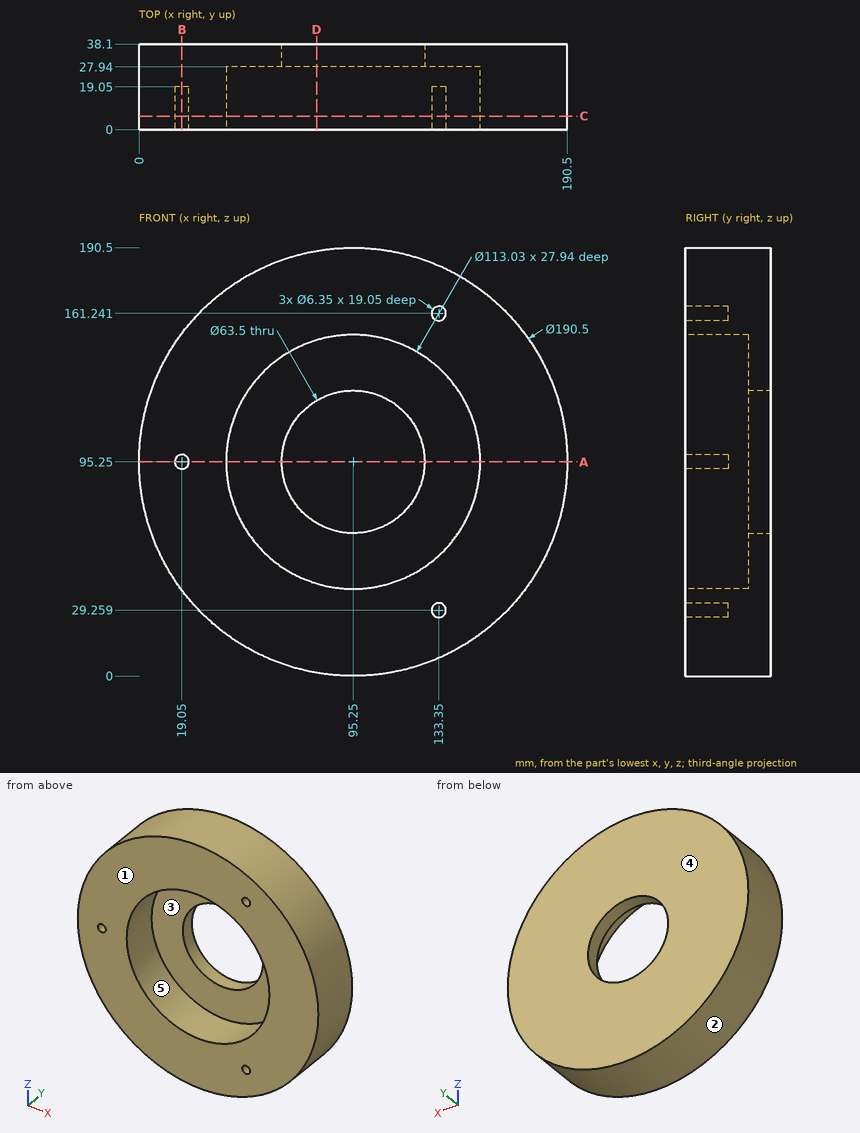
Source: three-view drawing plus pictorial views. Frame: mm from the lowest corner of the part. A direction names the side the tool comes from. Give positions to 0.01 mm unless a question says otherwise; leave off trailing zeros. Order: outer loops, then holes, each group sorted by start corner. A loop starts at its lowest first (then second) coordinate and runs counter-clockwise, first axis right, second up. Notation, with made-up numbers: (86.5, -36) - (118.5, -36) arc R27 cw to (118.5, -8) - close; hole circle Ø8 at (27.5, -23). An arc over 180 degrees is marked (long way). Answer as a JSON object with one key per item and string values. Group by question number.
Q1. Cut plane B-B, the plane x = 19.05. Output: boundary loops of the cut face in (y, z) (3 decimals).
Q2. Cut plane C-C, the plane y = 6. Count the separate pieces of the cut face and the enclosed holes in it, then the cut area to 3 significant figures.
Q3. Cut plane A-A, the plane z = 95.25. Output: boundary loops of the cut face in (x, y) (3 decimals).
Q4. Line query: probe 1 along X at (y, z) = (13, 95) (1 decimal); probe 2 along Z at (x, y) = (95.25, 33); probe 3 along Z at (x, y) = (133.35, 13.5). Output: solid intervals per line, ascending.
Q5. First-contact query: pin 1 Ø1.9 at (x, z) = (17.5, 95) entering from -Y; pin 2 Ø2 at (x, y) = (75, 16.5) entering from +Z; pin 3 Ø6 at (y, z) = (33.5, 28.5) entering from -X. Flat tips, straight axial feed; report the tip coordinate or a pass-through.
Q6. Mould query, pull axis Z, two halves, no side actions, for the marked faces 1, 2 and 3. Classes: pulls with the +Z half, pulls with the -Z half, needs draft (parallel to the pull), parting line crosses it, or undercut.
Q7. Cut plane D-D, the plane x = 79. Output: boundary loops of the cut face in (y, z).
Q8. Set-up query: the marked faces 4 and 5. Return all of +Z, -Z, +X, -X, +Y, -Y with unobstructed straight access to the full face (end or side cutting, diameter ignored); none if empty.
Results:
{
 "1": {"outline": "(0, 38.1) - (38.1, 38.1) - (38.1, 152.4) - (0, 152.4) - (0, 98.425) - (19.05, 98.425) - (19.05, 92.075) - (0, 92.075) - close"},
 "2": {"separate pieces": "1", "enclosed holes": "4", "area": "18,400 mm^2"},
 "3": {"outline": "(0, 0) - (15.875, 0) - (15.875, 19.05) - (22.225, 19.05) - (22.225, 0) - (38.735, 0) - (38.735, 27.94) - (63.5, 27.94) - (63.5, 38.1) - (0, 38.1) - close; (127, 27.94) - (151.765, 27.94) - (151.765, 0) - (190.5, 0) - (190.5, 38.1) - (127, 38.1) - close"},
 "4": {"probe 1": "0 to 15.9, 22.2 to 38.7, 151.8 to 190.5", "probe 2": "0 to 63.5, 127 to 190.5", "probe 3": "7.95 to 26.08, 32.43 to 53.51, 136.99 to 158.07, 164.42 to 182.55"},
 "5": {"pin 1": "y = 19.05", "pin 2": "z = 188.53", "pin 3": "x = 24.48"},
 "6": {"face 1": "needs draft", "face 2": "parting line crosses it", "face 3": "undercut"},
 "7": {"outline": "(0, 1.4) - (38.1, 1.4) - (38.1, 67.97) - (27.94, 67.97) - (27.94, 41.12) - (0, 41.12) - close; (0, 149.38) - (27.94, 149.38) - (27.94, 122.53) - (38.1, 122.53) - (38.1, 189.1) - (0, 189.1) - close"},
 "8": {"face 4": "+Z, -Z, +X, -X, +Y", "face 5": "-Y"}
}
